from build123d import *

# Parameters (mm, degrees)
F0_W     = 127
F0_H     = 50.8
F1_DEPTH = 38.1
F2_W     = 38.1
F2_H     = 50.8
F3_DEPTH = 25.4
F4_DEPTH = 38.1


with BuildPart() as f1:
    # F0 (on Top) → F1 (new body, symmetric)
    with BuildSketch(Plane.XY):
        Rectangle(F0_W, F0_H)
    extrude(amount=F1_DEPTH, both=True)

    # F2 (on face) → F3 (cut)
    with BuildSketch(Plane.XY.offset(38.1)):
        with Locations((-44.45, 0)):
            Rectangle(F2_W, F2_H)
        with Locations((44.45, 0)):
            Rectangle(F2_W, F2_H)
    extrude(amount=-F3_DEPTH, mode=Mode.SUBTRACT)

    # F2 (on face) → F4 (cut)
    with BuildSketch(Plane.XY.offset(38.1)):
        with Locations((-44.45, 0)):
            Rectangle(F2_W, F2_H)
        with Locations((44.45, 0)):
            Rectangle(F2_W, F2_H)
    extrude(amount=-F4_DEPTH, mode=Mode.SUBTRACT)


solid = f1.part
For this review, take the finished solid that the model builds, in its own axes (mm). A direction names the side the tool comes from. Round coordinates to 2 decimals unless told otherwise and drop trailing zeros. Order: outer loops, then holes, each group sorted by start corner. A loop starts at its lowest first (then second) coordinate and runs counter-clockwise, first axis right, second up. Notation, with made-up numbers: (81, -10.5) -> (120, -10.5) arc R14 ccw to (120, -5.5) -> close; hole circle Ø10 at (-7, 64.25). An arc over 180 degrees is marked (long way). Write item = value, one per line. Start each with the question number.
1) Tool access review of faces 1 (the face through (44, 0, 0)), 2 (the face through (-45, 0, 0)), 3 (the face through (-63.5, 0, -19)): name each direction out of +Z, -Z, +X, -X, +Y, -Y from which nothing blocks a thin tool from reaching the whole face with its end or side.
2) Take a section at C-C on x = 44.5. State the section outline as (y, z) points, plus the area to 3 significant figures.
3) Insertion check: pin 1 (11.5 mm diameter, centred on y = 8, z = 14, fed in from +X); pin 2 (19 mm diameter, centred on x = 43, y = 3.5, fed in from +Z); pin 3 (8 mm diameter, centred on y = -19, z = 7, fed in from -X). Each pin has a flat end and moves straight along its axis. Give the tip position at first contact, or say it passes through.
4) Take a section at A-A on y = -4.5. State the section outline as (x, z) points, plus the area to 3 significant figures.
5) To check wall thickness, follow line 1 (Z direction, x = 32.5, y = -11); line 2 (X direction, y = -10.5, z = 32). State the ranges of each line that lie inside material, in increasing order. Write a range as from..to.
6) Take a section at B-B on z = 23. State the section outline as (x, y) points.
Verdict:
q1.face_1 = +Z, +X, +Y, -Y
q1.face_2 = +Z, -X, +Y, -Y
q1.face_3 = +Z, -Z, -X, +Y, -Y
q2.outline = (-25.4, -38.1) -> (25.4, -38.1) -> (25.4, 0) -> (-25.4, 0) -> close
q2.area = 1,940 mm2
q3.pin_1 = 25.4
q3.pin_2 = 0
q3.pin_3 = -25.4
q4.outline = (-63.5, -38.1) -> (63.5, -38.1) -> (63.5, 0) -> (25.4, 0) -> (25.4, 38.1) -> (-25.4, 38.1) -> (-25.4, 0) -> (-63.5, 0) -> close
q4.area = 6,770 mm2
q5.line_1 = -38.1..0
q5.line_2 = -25.4..25.4
q6.outline = (-25.4, -25.4) -> (25.4, -25.4) -> (25.4, 25.4) -> (-25.4, 25.4) -> close
